```python
from build123d import *

# Parameters (mm, degrees)
F0_W     = 63.5
F0_H     = 27.94
F1_DEPTH = 66.675
F2_T     = -3.048
F4_DEPTH = 25.4


with BuildPart() as f1:
    # F0 (on Front) → F1 (new body)
    with BuildSketch(Plane.XZ):
        Rectangle(F0_W, F0_H)
    extrude(amount=F1_DEPTH)

    # F2
    f2_openings = [f1.faces().sort_by_distance(p)[0] for p in [
        (0, -33.3375, 13.97),
    ]]
    offset(amount=F2_T, openings=f2_openings)

    # F3 (on face) → F4 (cut)
    with BuildSketch(Plane(origin=(0, -63.627, 0), x_dir=(-1, 0, 0), z_dir=(0, 1, 0))):
        Polygon((12.7, -5.7555163684), (28.702, 13.97), (-28.702, 13.97), (-12.7, -5.7555163684), (0, -5.7555163684), align=None)
    extrude(amount=-F4_DEPTH, mode=Mode.SUBTRACT)


solid = f1.part
```
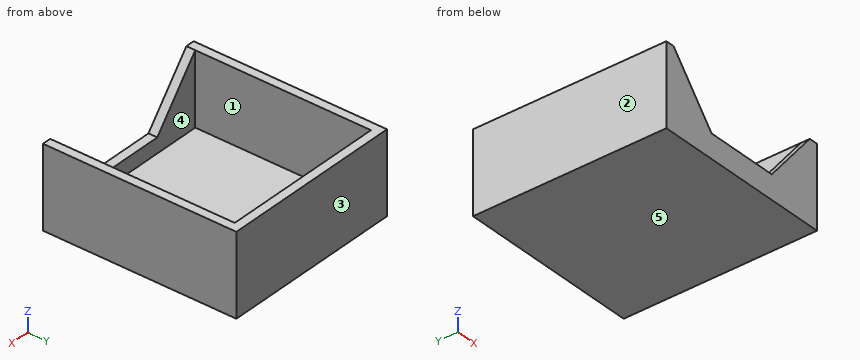
Design review of the part built by this model. Coordinates are the model's own, in mm. Face numbers are marked on the shaded views. A direction names the side the tool comes from. Coordinates: 2 decimals unless noted, no trailing zeros. Order: outer loops, then holes, each group sorted by start corner. A loop starts at its lowest first (then second) coordinate and runs counter-clockwise, first axis right, second up. Notation, with made-up numbers: (89, 24.5) - (144, 24.5) arc R17 ccw to (144, 43.5) - close; hole circle Ø9 at (69, 40.5). An arc over 180 degrees is marked (long way). One line per question, with ' | ' between items.
Q1. To check wall thickness, follow line 1 along X through (y, z) = (-36.5, -3.5); line 2 along Y through (x, z) = (-12, -7.5) (3 decimals); line 3 along Y through (x, z) = (-8, 2.25). State the ranges of each line that lie inside material, in increasing order.
Answer key:
line 1: x = -31.75 to -28.7, 28.7 to 31.75 | line 2: y = -66.675 to -63.627, -3.048 to 0 | line 3: y = -3.05 to 0
Q2. The part is to be moulded in two halves that separate along X. For the marked faces 1, 2 and 3, say which applies: +X half, -X half, draft (parallel to the pull), parting line (faces both ways), or undercut.
Answer key:
face 1: undercut | face 2: -X half | face 3: draft
Q3. Consider section A-A, the plane z = -7.75. Give the boundary of the cut face in (x, y) (3 decimals).
Answer key:
outline: (-31.75, -66.675) - (31.75, -66.675) - (31.75, 0) - (-31.75, 0) - close; hole (-28.702, -63.627) - (28.702, -63.627) - (28.702, -3.048) - (-28.702, -3.048) - close
Q4. Consider section B-B, the plane x = 8.5. Give the boundary of the cut face in (y, z) (3 decimals).
Answer key:
outline: (-66.675, -13.97) - (0, -13.97) - (0, 13.97) - (-3.048, 13.97) - (-3.048, -10.922) - (-63.627, -10.922) - (-63.627, -5.756) - (-66.675, -5.756) - close
Q5. Consider section C-C, the plane y = -24. Give the boundary of the cut face in (x, z), then the cut area to 3 significant figures.
Answer key:
outline: (-31.75, -13.97) - (31.75, -13.97) - (31.75, 13.97) - (28.7, 13.97) - (28.7, -10.92) - (-28.7, -10.92) - (-28.7, 13.97) - (-31.75, 13.97) - close | area: 345 mm2
Q6. For the marked faces 4 and 5, list the 3-axis set-ups (+Z, -Z, +X, -X, +Y, -Y) from which the entire face can be reached by the end or side of a thin tool; tool diameter is ignored.
Answer key:
face 4: +Z | face 5: -Z, +X, -X, +Y, -Y
Q7. Clearance check with flat-ended pins moving along their axes: pin 1 Ø12.5 at (x, z) = (10.5, 4) entering from -Y; pin 2 Ø2 at (x, y) = (22, -43) entering from +Z; pin 3 Ø2.5 at (x, y) = (-5, -64.5) entering from +Z. State where each tip first meets the part, or that it passes through.
Answer key:
pin 1: stops at y = -3.05 | pin 2: stops at z = -10.92 | pin 3: stops at z = -5.76
Q8. Consider section D-D, the plane z = 7. Give the boundary of the cut face in (x, y) (3 decimals).
Answer key:
outline: (-31.75, -66.675) - (-23.048, -66.675) - (-23.048, -63.627) - (-28.702, -63.627) - (-28.702, -3.048) - (28.702, -3.048) - (28.702, -63.627) - (23.048, -63.627) - (23.048, -66.675) - (31.75, -66.675) - (31.75, 0) - (-31.75, 0) - close
